The listing builds one solid part. Answer for the finished solid, in the listing's coordinates (mm). A direction names the side the tool comes from. Give positions to 0.01 mm unless a question says otherwise; leave off trailing zeros. Loops run counter-clockwise (first coordinate to the right, second up) from the corner with the lowest first, then second, coordinate; pieces in that order, holes last. Notation, with made-up numbers: M 75.25,22.25 L 97.25,22.25 A17 cw 97.25,36.25 Z; hole C 7.5,11.5 d8. An arc over 180 degrees is marked long. One line per item, written item: value. Start each with the question number.
Q1. A cutting plane is placed at A-A, the plane z = -9.5. Determine the outline of the cut face in (x, y), and give its area (3 significant figures).
Q2. A cutting plane is placed at C-C, the plane x = -63. Determine the outline of the cut face in (y, z).
Q3. Flat-ended cylindrical pins translate along their axes: pin 1 (10 mm diameter, centred on x = -35.5, y = -23, fed in from -Z); pin 2 (6.5 mm diameter, centred on x = -26.5, z = 4, fed in from +Y); pin 3 (4.5 mm diameter, centred on x = -62, z = -1, fed in from +Y); pin 4 (3 mm diameter, centred on y = -20.5, z = 5, fed in from -X). Find the tip coordinate at first contact, or state that the pin passes through.
Q4. For faces 4 (the flat face through (-25.054, -6, 0)), 5 (the flat face through (-60.991, -26, 0)), 6 (the flat face through (-27, -28.726, 0)), 7 (the flat face through (-65.73, -7, 0)), 8 (the flat face through (-60.153, -7, 0)), determine the directions among +Z, -Z, +X, -X, +Y, -Y from which every point of the face is accessible in a straight line to the end or side of a thin tool.
Q5. The mould has two halves that part along Y. Classify faces 1 (the flat face through (-27, -23.256, 0)), 2 (the flat face through (-27, -26, -13.276)), 3 (the flat face through (-63, -4.04, 0)): +Y half, -Y half, draft (parallel to the pull), parting line (faces both ways), or undercut.
Q6. Consider L1, parallel to X at y = -6.5, z = -2.5; L2, parallel to Y at x = -28, z = 5; L3, parallel to Z at x = -27, y = -21. Determine where each line is inside the solid, lowest interval first.
Q7. A cutting plane is placed at B-B, the plane y = -24.5. Determine the outline of the cut face in (x, z).
Q8. A cutting plane is placed at D-D, the plane x = -55. Determine the outline of the cut face in (y, z).
from build123d import *

# Parameters (mm, degrees)
F0_W     = 51.322882995
F0_H     = 4.9239350483
F1_DEPTH = 33.274
F2_W     = 4.1453018785
F2_H     = 5.1284935325
F3_DEPTH = 25.4
F4_W     = 4.7375038266
F4_H     = 5.470385775
F5_DEPTH = 25.4
F6_W     = 5.5771172047
F6_H     = 5.1148859784
F7_DEPTH = 25.4
F8_W     = 6.0726962984
F8_H     = 4.2278408073
F9_DEPTH = 25.4


with BuildPart() as f1:
    # F0 (on Front) → F1 (new body)
    with BuildSketch(Plane.XZ):
        with Locations((-45.2036233619, 14.5862386562)):
            Rectangle(F0_W, F0_H)
    extrude(amount=F1_DEPTH)

    # F2 (on face) → F3 (join)
    with BuildSketch(Plane(origin=(0, 0, 12.1242711321), x_dir=(1, 0, 0), z_dir=(0, 0, -1))):
        with Locations((-63.0641318858, 26.5037836507)):
            Rectangle(F2_W, F2_H)
    extrude(amount=F3_DEPTH)

    # F4 (on face) → F5 (join)
    with BuildSketch(Plane(origin=(0, 0, 12.1242711321), x_dir=(1, 0, 0), z_dir=(0, 0, -1))):
        with Locations((-27.434207499, 25.9909359738)):
            Rectangle(F4_W, F4_H)
    extrude(amount=F5_DEPTH)

    # F6 (on face) → F7 (join)
    with BuildSketch(Plane(origin=(0, 0, 12.1242711321), x_dir=(1, 0, 0), z_dir=(0, 0, -1))):
        with Locations((-62.9411712289, 6.5979263745)):
            Rectangle(F6_W, F6_H)
    extrude(amount=F7_DEPTH)

    # F8 (on face) → F9 (join)
    with BuildSketch(Plane(origin=(0, 0, 12.1242711321), x_dir=(1, 0, 0), z_dir=(0, 0, -1))):
        with Locations((-28.0904341489, 6.2653592322)):
            Rectangle(F8_W, F8_H)
    extrude(amount=F9_DEPTH)


solid = f1.part
Answer block:
1. outline: M -65.73,-9.16 L -60.15,-9.16 L -60.15,-4.04 L -65.73,-4.04 Z; M -65.14,-29.07 L -60.99,-29.07 L -60.99,-23.94 L -65.14,-23.94 Z; M -31.13,-8.38 L -25.05,-8.38 L -25.05,-4.15 L -31.13,-4.15 Z; M -29.8,-28.73 L -25.07,-28.73 L -25.07,-23.26 L -29.8,-23.26 Z
1. area: 101 mm^2
2. outline: M -33.27,12.12 L -29.07,12.12 L -29.07,-13.28 L -23.94,-13.28 L -23.94,12.12 L -9.16,12.12 L -9.16,-13.28 L -4.04,-13.28 L -4.04,12.12 L 0,12.12 L 0,17.05 L -33.27,17.05 Z
3. pin 1: z = 12.12
3. pin 2: y = -4.15
3. pin 3: y = -4.04
3. pin 4: through
4. face 4: -Z, +X, +Y, -Y
4. face 5: -Z, -Y
4. face 6: -Z, +X, -Y
4. face 7: -Z, -X, +Y, -Y
4. face 8: -Z, +Y, -Y
5. face 1: undercut
5. face 2: draft
5. face 3: +Y half
6. L1: -65.73 to -60.15, -31.13 to -25.05
6. L2: -28.73 to -23.26, -8.38 to -4.15
6. L3: 12.12 to 17.05
7. outline: M -70.87,12.12 L -65.14,12.12 L -65.14,-13.28 L -60.99,-13.28 L -60.99,12.12 L -29.8,12.12 L -29.8,-13.28 L -25.07,-13.28 L -25.07,12.12 L -19.54,12.12 L -19.54,17.05 L -70.87,17.05 Z
8. outline: M -33.27,12.12 L 0,12.12 L 0,17.05 L -33.27,17.05 Z
